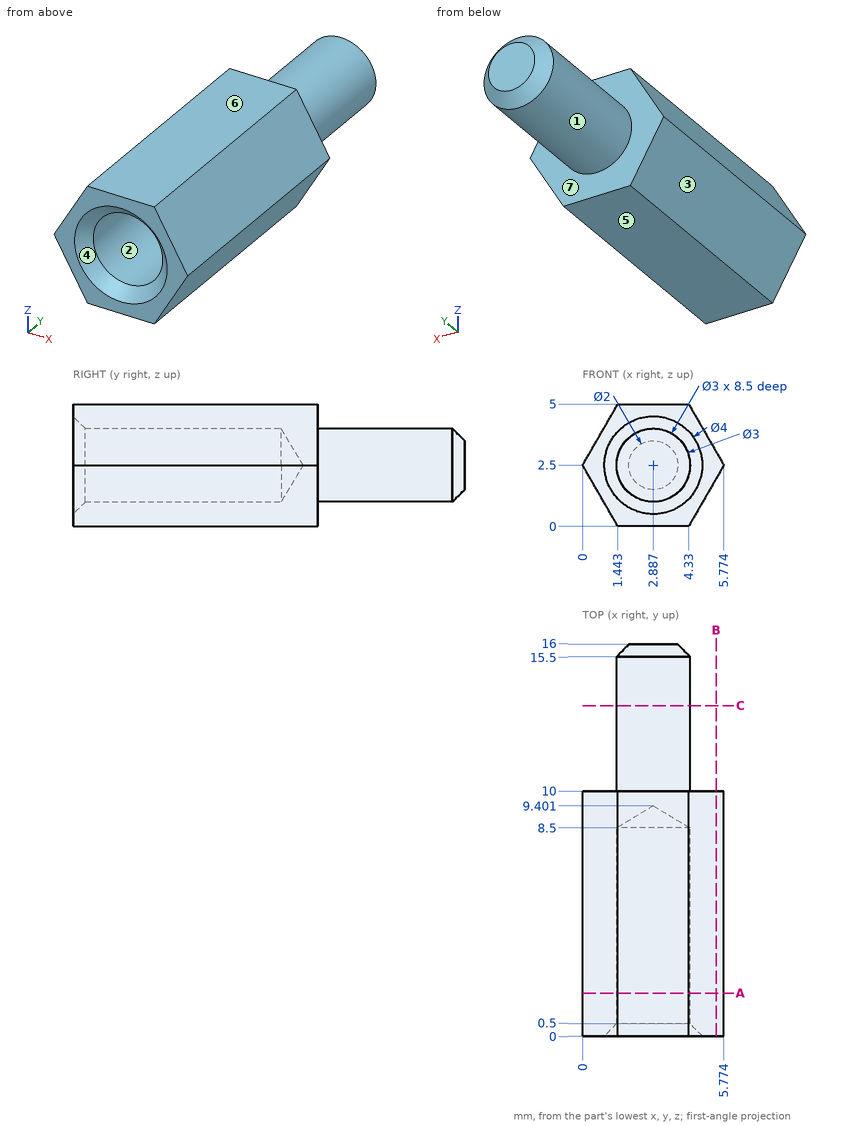
Answer from the drawing. Dimensions are ordinates in mm from the lowest x, y and z of the part. A direction names the side the tool comes from. Give positions to 0.01 mm unless a question says otherwise; leave off trailing zeros. Write each loop counter-clockwise with the first axis right and the second up, starting at its lowest first coordinate (ties: lowest second). Pieces come first, ordered by that corner, then holes. Notation, with made-up numbers: (33.25, 76.5) - (40.25, 76.5) arc R7 cw to (40.25, 85.5) - close; hole circle Ø1 at (-28, 76.5). An arc over 180 degrees is marked (long way). Answer in a Markdown table with one row per item. Add a question column.
Item 1: Find the intervals of material crossed by L1, parallel to Z at x = 2.95, y = 5; L2, parallel to Y at x = 1.5, z = 0.35; L3, parallel to Z at x = 2.4, y = 7, in increasing order.
Item 2: Section A-A, the plane y = 1.75 is taken. Write down the section's boundary in (x, z), and give its area (3 significant figures).
Item 3: Section C-C, the plane y = 13.5 is taken. Write down the section's boundary in (x, z).
Item 4: Determine the mould class of the marked faces 4, 5, 6 and 7 for opening direction Z: pulls with the +Z half, pulls with the -Z half, needs draft (parallel to the pull), parting line crosses it, or undercut.
Item 5: Flat-ended cylindrical pins translate along their axes: P1, Ø1, axis at y = 12.5, z = 1, coming from the -X side; P2, Ø2, axis at y = 11.5, z = 4, coming from the -X side; P3, Ø3, axis at x = 3, y = 13, coming from the +Z side. Find the tip coordinate at first contact, or state that the pin passes through.
Item 6: A tool of negligible diameter and unlimited length cuts with its end or side. For the marked faces 1, 2 and 3, from which of +Z, -Z, +X, -X, +Y, -Y can it reach the whole face along a straight path? Write none if from no direction.
Item 7: Section B-B, the plane x = 5.45 is taken. Write down the section's boundary in (y, z).
Recorded:
| question | item | result |
|---|---|---|
| 1 | L1 | z = 0 to 1, 4 to 5 |
| 1 | L2 | y = 0 to 10 |
| 1 | L3 | z = 0 to 1.08, 3.92 to 5 |
| 2 | outline | (0, 2.5) - (1.44, 0) - (4.33, 0) - (5.77, 2.5) - (4.33, 5) - (1.44, 5) - close; hole circle Ø3 at (2.89, 2.5) |
| 2 | area | 14.6 mm2 |
| 3 | outline | circle Ø3 at (2.89, 2.5) |
| 4 | face 4 | undercut |
| 4 | face 5 | pulls with the -Z half |
| 4 | face 6 | pulls with the +Z half |
| 4 | face 7 | needs draft |
| 5 | P1 | stops at x = 1.77 |
| 5 | P2 | stops at x = 1.47 |
| 5 | P3 | stops at z = 4 |
| 6 | face 1 | +Y |
| 6 | face 2 | -Y |
| 6 | face 3 | -Z, -X, +Y, -Y |
| 7 | outline | (0, 1.94) - (10, 1.94) - (10, 3.06) - (0, 3.06) - close |
